from build123d import *

# Parameters (mm, degrees)
CROQUIS1_R                 = 2
SALIENTE_EXTRUIR1_DEPTH    = 3.5
SALIENTE_EXTRUIR1_2_DEPTH  = 3.5
SALIENTE_EXTRUIR1_3_DEPTH  = 3.5
SALIENTE_EXTRUIR1_4_DEPTH  = 3.5
SALIENTE_EXTRUIR1_5_DEPTH  = 3.5
SALIENTE_EXTRUIR1_6_DEPTH  = 3.5
SALIENTE_EXTRUIR1_7_DEPTH  = 3.5
SALIENTE_EXTRUIR1_8_DEPTH  = 3.5
SALIENTE_EXTRUIR1_9_DEPTH  = 3.5
SALIENTE_EXTRUIR1_10_DEPTH = 3.5
SALIENTE_EXTRUIR1_11_DEPTH = 3.5
SALIENTE_EXTRUIR1_12_DEPTH = 3.5
SALIENTE_EXTRUIR1_13_DEPTH = 3.5
SALIENTE_EXTRUIR1_14_DEPTH = 3.5
SALIENTE_EXTRUIR1_15_DEPTH = 3.5
SALIENTE_EXTRUIR1_16_DEPTH = 3.5
CROQUIS3_R                 = 30
CROQUIS3_R_2               = 25
SALIENTE_EXTRUIR2_DEPTH    = 6
CROQUIS4_R                 = 1.52
CORTAR_EXTRUIR1_DEPTH      = 45.09081537


with BuildPart() as part:
    # Croquis1 → Saliente-Extruir1 (new, symmetric)
    with BuildSketch(Plane(origin=(0, 0, 0), x_dir=(1, 0, 0), z_dir=(0, 1, 0))):
        with Locations(Location((25, 0, 0), (0, 0, 270))):
            Circle(CROQUIS1_R)
    extrude(amount=SALIENTE_EXTRUIR1_DEPTH, both=True)



with BuildPart() as body_2:
    # Croquis1 → Saliente-Extruir1 2 (new, symmetric)
    with BuildSketch(Plane(origin=(0, 0, 0), x_dir=(1, 0, 0), z_dir=(0, 1, 0))):
        with Locations(Location((23.096988313, -9.567085809, 0), (0, 0, 270))):
            Circle(CROQUIS1_R)
    extrude(amount=SALIENTE_EXTRUIR1_2_DEPTH, both=True)


with BuildPart() as body_3:
    # Croquis1 → Saliente-Extruir1 3 (new, symmetric)
    with BuildSketch(Plane(origin=(0, 0, 0), x_dir=(1, 0, 0), z_dir=(0, 1, 0))):
        with Locations(Location((17.67766953, -17.67766953, 0), (0, 0, 270))):
            Circle(CROQUIS1_R)
    extrude(amount=SALIENTE_EXTRUIR1_3_DEPTH, both=True)


with BuildPart() as body_4:
    # Croquis1 → Saliente-Extruir1 4 (new, symmetric)
    with BuildSketch(Plane(origin=(0, 0, 0), x_dir=(1, 0, 0), z_dir=(0, 1, 0))):
        with Locations(Location((9.567085809, -23.096988313, 0), (0, 0, 270))):
            Circle(CROQUIS1_R)
    extrude(amount=SALIENTE_EXTRUIR1_4_DEPTH, both=True)


with BuildPart() as body_5:
    # Croquis1 → Saliente-Extruir1 5 (new, symmetric)
    with BuildSketch(Plane(origin=(0, 0, 0), x_dir=(1, 0, 0), z_dir=(0, 1, 0))):
        with Locations(Location((0, -25, 0), (0, 0, 270))):
            Circle(CROQUIS1_R)
    extrude(amount=SALIENTE_EXTRUIR1_5_DEPTH, both=True)


with BuildPart() as body_6:
    # Croquis1 → Saliente-Extruir1 6 (new, symmetric)
    with BuildSketch(Plane(origin=(0, 0, 0), x_dir=(1, 0, 0), z_dir=(0, 1, 0))):
        with Locations(Location((-9.567085809, -23.096988313, 0), (0, 0, 270))):
            Circle(CROQUIS1_R)
    extrude(amount=SALIENTE_EXTRUIR1_6_DEPTH, both=True)


with BuildPart() as body_7:
    # Croquis1 → Saliente-Extruir1 7 (new, symmetric)
    with BuildSketch(Plane(origin=(0, 0, 0), x_dir=(1, 0, 0), z_dir=(0, 1, 0))):
        with Locations(Location((-17.67766953, -17.67766953, 0), (0, 0, 270))):
            Circle(CROQUIS1_R)
    extrude(amount=SALIENTE_EXTRUIR1_7_DEPTH, both=True)


with BuildPart() as body_8:
    # Croquis1 → Saliente-Extruir1 8 (new, symmetric)
    with BuildSketch(Plane(origin=(0, 0, 0), x_dir=(1, 0, 0), z_dir=(0, 1, 0))):
        with Locations(Location((-23.096988313, -9.567085809, 0), (0, 0, 270))):
            Circle(CROQUIS1_R)
    extrude(amount=SALIENTE_EXTRUIR1_8_DEPTH, both=True)


with BuildPart() as body_9:
    # Croquis1 → Saliente-Extruir1 9 (new, symmetric)
    with BuildSketch(Plane(origin=(0, 0, 0), x_dir=(1, 0, 0), z_dir=(0, 1, 0))):
        with Locations(Location((-25, 0, 0), (0, 0, 270))):
            Circle(CROQUIS1_R)
    extrude(amount=SALIENTE_EXTRUIR1_9_DEPTH, both=True)


with BuildPart() as body_10:
    # Croquis1 → Saliente-Extruir1 10 (new, symmetric)
    with BuildSketch(Plane(origin=(0, 0, 0), x_dir=(1, 0, 0), z_dir=(0, 1, 0))):
        with Locations(Location((-23.096988313, 9.567085809, 0), (0, 0, 270))):
            Circle(CROQUIS1_R)
    extrude(amount=SALIENTE_EXTRUIR1_10_DEPTH, both=True)


with BuildPart() as body_11:
    # Croquis1 → Saliente-Extruir1 11 (new, symmetric)
    with BuildSketch(Plane(origin=(0, 0, 0), x_dir=(1, 0, 0), z_dir=(0, 1, 0))):
        with Locations(Location((-17.67766953, 17.67766953, 0), (0, 0, 270))):
            Circle(CROQUIS1_R)
    extrude(amount=SALIENTE_EXTRUIR1_11_DEPTH, both=True)


with BuildPart() as body_12:
    # Croquis1 → Saliente-Extruir1 12 (new, symmetric)
    with BuildSketch(Plane(origin=(0, 0, 0), x_dir=(1, 0, 0), z_dir=(0, 1, 0))):
        with Locations(Location((-9.567085809, 23.096988313, 0), (0, 0, 270))):
            Circle(CROQUIS1_R)
    extrude(amount=SALIENTE_EXTRUIR1_12_DEPTH, both=True)


with BuildPart() as body_13:
    # Croquis1 → Saliente-Extruir1 13 (new, symmetric)
    with BuildSketch(Plane(origin=(0, 0, 0), x_dir=(1, 0, 0), z_dir=(0, 1, 0))):
        with Locations(Location((0, 25, 0), (0, 0, 270))):
            Circle(CROQUIS1_R)
    extrude(amount=SALIENTE_EXTRUIR1_13_DEPTH, both=True)


with BuildPart() as body_14:
    # Croquis1 → Saliente-Extruir1 14 (new, symmetric)
    with BuildSketch(Plane(origin=(0, 0, 0), x_dir=(1, 0, 0), z_dir=(0, 1, 0))):
        with Locations(Location((9.567085809, 23.096988313, 0), (0, 0, 270))):
            Circle(CROQUIS1_R)
    extrude(amount=SALIENTE_EXTRUIR1_14_DEPTH, both=True)


with BuildPart() as body_15:
    # Croquis1 → Saliente-Extruir1 15 (new, symmetric)
    with BuildSketch(Plane(origin=(0, 0, 0), x_dir=(1, 0, 0), z_dir=(0, 1, 0))):
        with Locations(Location((17.67766953, 17.67766953, 0), (0, 0, 270))):
            Circle(CROQUIS1_R)
    extrude(amount=SALIENTE_EXTRUIR1_15_DEPTH, both=True)


with BuildPart() as body_16:
    # Croquis1 → Saliente-Extruir1 16 (new, symmetric)
    with BuildSketch(Plane(origin=(0, 0, 0), x_dir=(1, 0, 0), z_dir=(0, 1, 0))):
        with Locations(Location((23.096988313, 9.567085809, 0), (0, 0, 270))):
            Circle(CROQUIS1_R)
    extrude(amount=SALIENTE_EXTRUIR1_16_DEPTH, both=True)


with BuildPart() as part_1:
    add(part.part)

    add(body_2.part)  # Saliente-Extruir2 merges body 2

    add(body_3.part)  # Saliente-Extruir2 merges body 3

    add(body_4.part)  # Saliente-Extruir2 merges body 4

    add(body_5.part)  # Saliente-Extruir2 merges body 5

    add(body_6.part)  # Saliente-Extruir2 merges body 6

    add(body_7.part)  # Saliente-Extruir2 merges body 7

    add(body_8.part)  # Saliente-Extruir2 merges body 8

    add(body_9.part)  # Saliente-Extruir2 merges body 9

    add(body_10.part)  # Saliente-Extruir2 merges body 10

    add(body_11.part)  # Saliente-Extruir2 merges body 11

    add(body_12.part)  # Saliente-Extruir2 merges body 12

    add(body_13.part)  # Saliente-Extruir2 merges body 13

    add(body_14.part)  # Saliente-Extruir2 merges body 14

    add(body_15.part)  # Saliente-Extruir2 merges body 15

    add(body_16.part)  # Saliente-Extruir2 merges body 16
    # Croquis3 → Saliente-Extruir2 (add, symmetric)
    with BuildSketch(Plane(origin=(0, 0, 0), x_dir=(1, 0, 0), z_dir=(0, 1, 0))):
        with Locations(Location((0, 0, 0), (0, 0, 270))):
            Circle(CROQUIS3_R)
        with Locations(Location((0, 0, 0), (0, 0, 270))):
            Circle(CROQUIS3_R_2, mode=Mode.SUBTRACT)
    extrude(amount=SALIENTE_EXTRUIR2_DEPTH, both=True)

    # Croquis4 → Cortar-Extruir1 (cut, through all)
    with BuildSketch(Plane(origin=(0, 6, 0), x_dir=(1, 0, 0), z_dir=(0, 1, 0))):
        with Locations(Location((27.5, 0, 0), (0, 0, 270))):
            Circle(CROQUIS4_R)
        with Locations(Location((17.145969551, -21.500365768, 0), (0, 0, 270))):
            Circle(CROQUIS4_R)
        with Locations(Location((-6.119325684, -26.810517585, 0), (0, 0, 270))):
            Circle(CROQUIS4_R)
        with Locations(Location((-24.776643867, -11.931802826, 0), (0, 0, 270))):
            Circle(CROQUIS4_R)
        with Locations(Location((-24.776643867, 11.931802826, 0), (0, 0, 270))):
            Circle(CROQUIS4_R)
        with Locations(Location((-6.119325684, 26.810517585, 0), (0, 0, 270))):
            Circle(CROQUIS4_R)
        with Locations(Location((17.145969551, 21.500365768, 0), (0, 0, 270))):
            Circle(CROQUIS4_R)
    extrude(amount=-CORTAR_EXTRUIR1_DEPTH, mode=Mode.SUBTRACT)


solid = part_1.part
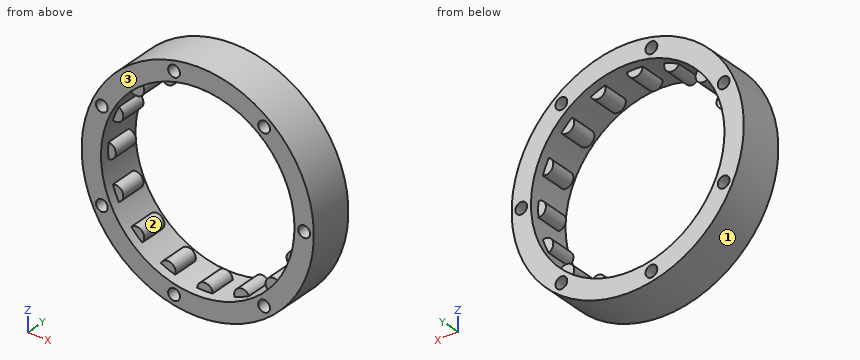
Design review of the part built by this model. Coordinates are the model's own, in mm. Face numbers are marked on the shaded views. Round coordinates to 2 decimals unless told otherwise and drop trailing zeros. Write each loop counter-clockwise with the first axis right and the second up, starting at its lowest first coordinate (ties: lowest second). Pieces come first, ordered by that corner, then holes. Notation, with made-up numbers: (-4.5, -25.75) - (20.5, -25.75) arc R16 ccw to (20.5, 2.25) - close; hole circle Ø8 at (73, 57). An arc over 180 degrees is marked (long way). Return JSON: item names as keys, results as strings. Group by question number.
Item 1: We need section D-D on y = -1. Give the number of separate pieces and of enclosed holes in the cut face, and give its area (3 significant figures).
Item 2: We need section A-A on x = 0. Write out the cut boundary in (y, z), and give its area (3 significant figures).
Item 3: The part is to be moulded in two halves that separate along Z. For the marked faces 1, 2 and 3, say which applies: pulls with the +Z half, pulls with the -Z half, needs draft (parallel to the pull), parting line crosses it, or undercut.
Item 4: We need section B-B on z = 0. Write out the cut boundary in (x, y).
Item 5: We need section C-C on x = -13.5. Write out the cut boundary in (y, z).
Item 6: For probe 1 along X at (y, z) = (2.75, 0); probe 2 along X at (y, z) = (-2.5, -21.5); probe 3 along Z at (x, y) = (-26, 2.25), list the stretches that pass through material, from the lowest coordinate up. Write a range as [from, to].
Item 7: Insertion check: P1, Ø5, axis at x = 19, y = 2, coming from the +Z side; P2, Ø5, axis at x = -22, y = 3.5, coming from the -Z side; P3, Ø4, axis at x = 18, y = -3, coming from the -Z side. Each pin has a flat end and moves straight along its axis. Give the tip position at first contact, or say it passes through.
Model answer:
{
 "1": {"separate pieces": "1", "enclosed holes": "8", "area": "912 mm²"},
 "2": {"outline": "(-6, -30) - (6, -30) - (6, -25) - (3.5, -25) - (3.5, -23) - (-3.5, -23) - (-3.5, -25) - (-6, -25) - close; (-6, 25) - (-3.5, 25) - (-3.5, 23) - (3.5, 23) - (3.5, 25) - (6, 25) - (6, 30) - (-6, 30) - close", "area": "148 mm²"},
 "3": {"face 1": "parting line crosses it", "face 2": "undercut", "face 3": "needs draft"},
 "4": {"outline": "(-30, -6) - (-25, -6) - (-25, -3.5) - (-23, -3.5) - (-23, 3.5) - (-25, 3.5) - (-25, 6) - (-30, 6) - close; (23, -3.5) - (25, -3.5) - (25, -6) - (25.98, -6) - (25.98, 6) - (25, 6) - (25, 3.5) - (23, 3.5) - close; (29.02, -6) - (30, -6) - (30, 6) - (29.02, 6) - close"},
 "5": {"outline": "(-6, -26.79) - (6, -26.79) - (6, -21.04) - (-6, -21.04) - close; (-6, 21.04) - (6, 21.04) - (6, 26.79) - (-6, 26.79) - close"},
 "6": {"probe 1": "x = [-30, -23], [23, 25.98], [29.02, 30]", "probe 2": "x = [-20.92, -12.76], [-10.77, -8.36], [8.36, 10.77], [12.76, 15.63], [18.67, 20.92]", "probe 3": "z = [-14.97, -12.83], [-11.03, 11.03], [12.83, 14.97]"},
 "7": {"P1": "stops at z = 25.05", "P2": "stops at z = -22.8", "P3": "stops at z = -25.38"}
}
